Autodesk Inventor part; units mm, degrees
ref_plane "Work Plane2" through (0, 0, 0) normal (0, 0, 1) x (1, 0, 0)
ref_plane "YZ Plane" through (0, 0, 0) normal (1, 0, 0) x (0, 1, 0)
ref_plane "XZ Plane" through (0, 0, 0) normal (0, 1, 0) x (-1, 0, 0)
ref_plane "Work Plane2" through (0, 0, 0) normal (0, 0, 1) x (1, 0, 0)
sketch "Sketch1" plane through (0, 0, 0) normal (0, 0, 1) x (1, 0, 0)
  line L0 (180, 126) -> (180, 200)
  arc A0 (180, 200) -> (175, 205) centre (175, 200) ccw
  line L1 (175, 205) -> (-174, 205)
  line L2 (-174, -368) -> (-174, 205)
  line L3 (-156, -368) -> (-174, -368)
  arc A1 (-153, -371) -> (-156, -368) centre (-156, -371) ccw
  line L4 (-153, -403) -> (-153, -371)
  arc A2 (-156, -406) -> (-153, -403) centre (-156, -403) ccw
  line L5 (-180, -406) -> (-156, -406)
  line L6 (-180, -406) -> (-180, -480)
  arc A3 (-180, -480) -> (-175, -485) centre (-175, -480) ccw
  line L7 (-175, -485) -> (174, -485)
  line L8 (174, 88) -> (174, -485)
  line L9 (156, 88) -> (174, 88)
  arc A4 (153, 91) -> (156, 88) centre (156, 91) ccw
  line L10 (153, 123) -> (153, 91)
  arc A5 (156, 126) -> (153, 123) centre (156, 123) ccw
  line L11 (180, 126) -> (156, 126)
  circle A6 centre (0, 0) radius 135
  circle A7 centre (82.55, 185) radius 3
  circle A8 centre (-82.55, 185) radius 3
  circle A9 centre (82.55, -460) radius 3
  circle A10 centre (-82.55, -460) radius 3
  line L12 (-149.5, -195) -> (-149.5, -395)
  arc A11 (-149.5, -395) -> (-110, -434.5) centre (-110, -395) ccw
  line L13 (-110, -434.5) -> (110, -434.5)
  arc A12 (110, -434.5) -> (149.5, -395) centre (110, -395) ccw
  line L14 (149.5, -395) -> (149.5, -195)
  arc A13 (149.5, -195) -> (110, -155.5) centre (110, -195) ccw
  line L15 (110, -155.5) -> (-110, -155.5)
  arc A14 (-110, -155.5) -> (-149.5, -195) centre (-110, -195) ccw
  line L16 (40, -245) -> (-40, -245)
  line L17 (-50, -255) -> (-50, -355)
  line L18 (-40, -365) -> (40, -365)
  line L19 (50, -355) -> (50, -255)
  arc A15 (-40, -245) -> (-50, -255) centre (-40, -255) ccw
  arc A16 (50, -255) -> (40, -245) centre (40, -255) ccw
  arc A17 (40, -365) -> (50, -355) centre (40, -355) ccw
  arc A18 (-50, -355) -> (-40, -365) centre (-40, -355) ccw
  point P0 (115, -175)
  point P1 (-50, -365)
  point P2 (-50, -245)
  point P3 (50, -365)
  dimension "d1" = 100
  dimension "d2" = 120
  dimension "d3" = 10
extrude "Extrusion1" add sketch "Sketch1" along normal blind 6.35 contours A14 L15 A13 L14 A12 L13 A11 L12
sketch "Sketch2" plane through (0, 0, 6.35) normal (0, 0, 1) x (1, 0, 0)
  line L0 (180, 126) -> (180, 200)
  arc A0 (180, 200) -> (175, 205) centre (175, 200) ccw
  line L1 (175, 205) -> (-174, 205)
  line L2 (-174, -368) -> (-174, 205)
  line L3 (-156, -368) -> (-174, -368)
  arc A1 (-153, -371) -> (-156, -368) centre (-156, -371) ccw
  line L4 (-153, -403) -> (-153, -371)
  arc A2 (-156, -406) -> (-153, -403) centre (-156, -403) ccw
  line L5 (-180, -406) -> (-156, -406)
  line L6 (-180, -406) -> (-180, -480)
  arc A3 (-180, -480) -> (-175, -485) centre (-175, -480) ccw
  line L7 (-175, -485) -> (174, -485)
  line L8 (174, 88) -> (174, -485)
  line L9 (156, 88) -> (174, 88)
  arc A4 (153, 91) -> (156, 88) centre (156, 91) ccw
  line L10 (153, 123) -> (153, 91)
  arc A5 (156, 126) -> (153, 123) centre (156, 123) ccw
  line L11 (180, 126) -> (156, 126)
  circle A6 centre (0, 0) radius 135
  circle A7 centre (-140, -217) radius 2
  circle A8 centre (-140, -269) radius 2
  circle A9 centre (-140, -321) radius 2
  circle A10 centre (-140, -373) radius 2
  circle A11 centre (-84, -425) radius 2
  circle A12 centre (-28, -425) radius 2
  circle A13 centre (28, -425) radius 2
  circle A14 centre (84, -425) radius 2
  circle A15 centre (140, -373) radius 2
  circle A16 centre (140, -321) radius 2
  circle A17 centre (140, -269) radius 2
  circle A18 centre (140, -217) radius 2
  circle A19 centre (84, -165) radius 2
  circle A20 centre (28, -165) radius 2
  circle A21 centre (-28, -165) radius 2
  circle A22 centre (-84, -165) radius 2
  line L12 (-130, -190) -> (-130, -400)
  arc A23 (-115, -175) -> (-130, -190) centre (-115, -190) ccw
  line L13 (115, -175) -> (-115, -175)
  arc A24 (130, -190) -> (115, -175) centre (115, -190) ccw
  line L14 (130, -400) -> (130, -190)
  arc A25 (115, -415) -> (130, -400) centre (115, -400) ccw
  line L15 (-115, -415) -> (115, -415)
  arc A26 (-130, -400) -> (-115, -415) centre (-115, -400) ccw
  circle A27 centre (82.55, 185) radius 3
  circle A28 centre (-82.55, 185) radius 3
  circle A29 centre (82.55, -460) radius 3
  circle A30 centre (-82.55, -460) radius 3
hole "Hole1" at (-140, -217, 6.35) at (-84, -165, 6.35) at (-28, -165, 6.35) at (28, -165, 6.35) at (84, -165, 6.35) at (-140, -269, 6.35) at (-140, -321, 6.35) at (-140, -373, 6.35) at (-84, -425, 6.35) at (-28, -425, 6.35) at (28, -425, 6.35) at (84, -425, 6.35) at (140, -373, 6.35) at (140, -321, 6.35) at (140, -269, 6.35) at (140, -217, 6.35) direction (0, 0, -1) diameter 5.5 end through all counterbore diameter 12.24 counterbore depth 2
sketch "Sketch3" plane through (0, 0, 6.35) normal (0, 0, 1) x (1, 0, 0)
  point P0 (0, 0)
  point P1 (-65, -305)
  point P2 (-65, -260)
  point P3 (-65, -350)
  point P4 (65, -305)
  point P5 (65, -260)
  point P6 (65, -350)
  point P7 (-20, -230)
  point P8 (20, -230)
  point P9 (-20, -380)
  point P10 (20, -380)
  dimension "d18" = 45
  dimension "d19" = 45
  dimension "d22" = 45
  dimension "d23" = 45
hole "Hole2" at (-65, -305, 6.35) at (-65, -260, 6.35) at (-65, -350, 6.35) at (65, -305, 6.35) at (65, -260, 6.35) at (65, -350, 6.35) at (-20, -230, 6.35) at (20, -230, 6.35) at (-20, -380, 6.35) at (20, -380, 6.35) direction (0, 0, -1) diameter 3.4587 depth 10.8 tip angle 118
sketch "Sketch4" plane through (0, 0, 6.35) normal (0, 0, 1) x (1, 0, 0)
  line L0 (100, -195) -> (-100, -195)
  line L1 (-100, -195) -> (-100, -395)
  line L2 (-100, -395) -> (100, -395)
  line L3 (100, -395) -> (100, -195)
  line L4 (0, 0) -> (0, -590.9398)
  line L5 (149.5, -395) -> (149.5, -195)
  line L6 (149.5, -295) -> (-173.2004, -295)
  line L7 (-40, -245) -> (40, -245)
  point P0 (0, -245)
  dimension "d46" = 200
  dimension "d47" = 200
  dimension "d48" = 100
  dimension "d49" = 100
extrude "Extrusion2" cut sketch "Sketch4" against normal blind 10
properties part number "Reducer Plate" material "Aluminum 6061"
The listing builds one solid part. Answer for the finished solid, in the listing's coordinates (mm). A direction names the side the tool comes from. Give positions to 0.01 mm unless a question says otherwise; leave off trailing zeros. Write each loop counter-clockwise with the first axis right and the second up, starting at its lowest first coordinate (ties: lowest second). Pieces come first, ordered by that corner, then holes. Notation, with made-up numbers: M 25.5,-15 L 29.5,-15 A19 cw 29.5,-10 Z; hole C -7,39 d7. An arc over 180 degrees is marked long. Write each question's results on one line, items separated by ' | '.
Q1. Section B-B, the plane y = -390 is taken. Write down the section's boundary in (x, z).
Output values:
outline: M -149.5,0 L -100,0 L -100,6.35 L -149.5,6.35 Z; M 100,0 L 149.5,0 L 149.5,6.35 L 100,6.35 Z
Q2. Flat-ended cylindrical pins translate along their axes: P1, Ø6.5, axis at x = -28, y = -425, coming from the +Z side; P2, Ø19.5, axis at x = 140, y = -373, coming from the -Z side; P3, Ø1.5, axis at x = 119, z = 3.5, coming from the +Y side. Find the tip coordinate at first contact, or state that the pin passes through.
Output values:
P1: z = 4.35 | P2: z = 0 | P3: y = -156.37
Q3. Section C-C, the plane x = -46 is taken. Write down the section's boundary in (y, z), then the cut area to 3 significant figures.
Output values:
outline: M -434.5,0 L -395,0 L -395,6.35 L -434.5,6.35 Z; M -195,0 L -155.5,0 L -155.5,6.35 L -195,6.35 Z | area: 502 mm2
Q4. Consider L1, parallel to Y at x = -84, z = 5.8; L2, parallel to Y at x = 84, z = 3; L3, parallel to X at y = -321, z = 5.25. Determine where each line is inside the solid, lowest interval first. Write a range as from..to.
Output values:
L1: -434.5..-431.12, -418.88..-395, -195..-171.12, -158.88..-155.5 | L2: -434.5..-427.75, -422.25..-395, -195..-167.75, -162.25..-155.5 | L3: -149.5..-146.12, -133.88..-100, 100..133.88, 146.12..149.5
Q5. For a pull along X with two mould halves and no side action, classify faces 1 (the cylindrical face through (-137.62, -423.24, 3.13)), 2 (the flat face through (-2, -434.5, 3)), 3 (the cylindrical face through (-140.269, -262.886, 5.336)) as released by +X, released by -X, zero draft, split by the parting line, or undercut.
Output values:
face 1: released by -X | face 2: zero draft | face 3: undercut
Q6. Section A-A, the plane z = 2.5 is taken. Count the separate pieces of the cut face and the enclosed holes in it, then the cut area to 3 significant figures.
Output values:
separate pieces: 1 | enclosed holes: 17 | area: 41,700 mm2
Q7. A tool of negligible diameter and unlimited length cuts with its end or side. For faces 4 (the cylindrical face through (-84.269, -158.886, 5.336)), 5 (the cylindrical face through (-138.24, -167.38, 3.13)), from which of +Z, -Z, +X, -X, +Y, -Y can it reach the whole face along a straight path? Write none if from no direction.
Output values:
face 4: +Z | face 5: +Z, -Z, -X, +Y
